from build123d import *

# Parameters (mm, degrees)
EXTRUDE1_DEPTH                      = 19.05
EXTRUDE1_DEPTH_BACK                 = 19.05
F_6_CLEARANCE_HOLE1_D               = 3.7973
F_6_CLEARANCE_HOLE1_DEPTH           = 6.35
F_6_CLEARANCE_HOLE1_TIP             = 1.140824014
F_6_CLEARANCE_HOLE1_ON_FACE_2_D     = 3.7973
F_6_CLEARANCE_HOLE1_ON_FACE_2_DEPTH = 6.35
F_6_CLEARANCE_HOLE1_ON_FACE_2_TIP   = 1.140824014
SKETCH3_W                           = 15.875
SKETCH3_H                           = 9.525
CUT_EXTRUDE1_DEPTH                  = 4.175
CHAMFER1_SIZE                       = 5.08


with BuildPart() as part:
    # Sketch1 → Extrude1 (new body, two sides)
    with BuildSketch(Plane(origin=(0, 0, 0), x_dir=(0, 0, -1), z_dir=(1, 0, 0))) as extrude1_sk:
        Polygon((-3.175, 9.525), (-3.175, -3.175), (9.525, -3.175), (9.525, 0), (0, 0), (0, 9.525), align=None)
    extrude(amount=EXTRUDE1_DEPTH)
    extrude(extrude1_sk.sketch, amount=-EXTRUDE1_DEPTH_BACK)

    # 6 Clearance Hole1
    with Locations(Plane(origin=(6.35, 0, -4.7625), x_dir=(0, 0, 1), z_dir=(0, 1, 0))):
        with Locations((0, 0), (0, -12.7)):
            Hole(F_6_CLEARANCE_HOLE1_D / 2, depth=F_6_CLEARANCE_HOLE1_DEPTH)
            with Locations((0, 0, -(F_6_CLEARANCE_HOLE1_DEPTH + F_6_CLEARANCE_HOLE1_TIP / 2))):  # 118° drill point
                Cone(0, F_6_CLEARANCE_HOLE1_D / 2, F_6_CLEARANCE_HOLE1_TIP, mode=Mode.SUBTRACT)

    # 6 Clearance Hole1 on face 2
    with Locations(Plane(origin=(3.175, 4.826, 0), x_dir=(-1, 0, 0), z_dir=(0, 0, -1))):
        with Locations((0, 0), (-9.525, 0)):
            Hole(F_6_CLEARANCE_HOLE1_ON_FACE_2_D / 2, depth=F_6_CLEARANCE_HOLE1_ON_FACE_2_DEPTH)
            with Locations((0, 0, -(F_6_CLEARANCE_HOLE1_ON_FACE_2_DEPTH + F_6_CLEARANCE_HOLE1_ON_FACE_2_TIP / 2))):  # 118° drill point
                Cone(0, F_6_CLEARANCE_HOLE1_ON_FACE_2_D / 2, F_6_CLEARANCE_HOLE1_ON_FACE_2_TIP, mode=Mode.SUBTRACT)

    # Sketch3 → Cut-Extrude1 (cut, through all)
    with BuildSketch(Plane(origin=(0, 0, 0), x_dir=(-1, 0, 0), z_dir=(0, 0, -1))):
        with Locations((11.1125, 4.7625)):
            Rectangle(SKETCH3_W, SKETCH3_H)
    extrude(amount=-CUT_EXTRUDE1_DEPTH, mode=Mode.SUBTRACT)

    # Chamfer1
    chamfer1_edges = [part.edges().sort_by_distance(p)[0] for p in [
        (19.05, -1.5875, -9.525),
        (-19.05, -1.5875, -9.525),
        (19.05, 9.525, 1.5875),
        (-3.175, 9.525, 1.5875),
    ]]
    chamfer(chamfer1_edges, length=CHAMFER1_SIZE)


solid = part.part
For this review, take the finished solid that the model builds, in its own axes (mm). A direction names the side the tool comes from. Give positions to 0.01 mm unless a question says otherwise; leave off trailing zeros. Loops run counter-clockwise (first coordinate to the right, second up) from the corner with the lowest first, then second, coordinate; pieces in that order, holes last. Notation, with made-up numbers: M 68.5,25.25 L 81.5,25.25 A22 cw 81.5,60.25 Z; hole C 15,-34.75 d4. An arc over 180 degrees is marked long. Put each result on its own line as item: value. Start each with the question number.
(1) Wall thickness on L1, parallel to Y at x = 12.7, z = 1.15 (3 decimals); L2, parallel to X at y = 6.5, z = 0.25 (3 decimals); L3, parallel to Y at x = 14, z = -6.25 (3 decimals): over which ranges is each line inside the solid? List them lowest first.
(2) The part is to be moulded in two halves that separate along X. For faces 1 (the cylindrical face through (4.93, 4.1, 1.61)), 2 (the flat face through (16.546, -1.61, -6.949)), 3 (the flat face through (-3.175, 2, 2)), say which applies: +X half, -X half, draft (parallel to the pull), parting line (faces both ways), or undercut.
(3) Machinability: for faces 4 (the flat face through (8, 5, 0)), 5 (the flat face through (5, 2, 3.175)), which of the approach directions +Z, -Z, +X, -X, +Y, -Y give a long, thin tool a straight path to every point of the face, cutting with its end or side? Answer none if there is none.
(4) Add section C-C, the plane z = -0.75. Write out the cut boundary in (x, y) (3 decimals).
(5) For pin 1 (3 mm diameter, centred on x = 10, y = 5, fed in from -Z); pin 2 (2.5 mm diameter, centred on y = 1.5, z = 2.5, fed in from -X) (3 decimals), all flat-tipped, find the tip position at first contact; note any pin that passes through.
(6) Add section B-B, the plane x = 0. Write out the cut boundary in (y, z) (3 decimals), then the cut area to 3 significant figures.
(7) Add section A-A, the plane x = 12.7. Write out the cut boundary in (y, z) (3 decimals).
(8) Add section D-D, the plane x = -6.35. Write out the cut boundary in (y, z) (3 decimals).
Result:
1. L1: y = -3.175 to 2.927, 6.725 to 9.525
1. L2: x = -1.12 to 2.279, 4.071 to 11.804, 13.596 to 16.995
1. L3: y = -3.175 to 0
2. face 1: undercut
2. face 2: +X half
2. face 3: -X half
3. face 4: -Z, +X, -X, +Y
3. face 5: +Z, +X, -X, +Y, -Y
4. outline: M -19.05,-3.175 L 19.05,-3.175 L 19.05,0 L -19.05,0 Z
5. pin 1: stops at z = 0
5. pin 2: stops at x = -3.175
6. outline: M -3.175,-9.525 L 0,-9.525 L 0,0 L 7.62,0 L 7.62,3.175 L -3.175,3.175 Z
6. area: 64.5 mm^2
7. outline: M -3.175,-9.525 L 0,-9.525 L 0,0 L 2.927,0 L 2.927,3.175 L -3.175,3.175 Z; M 6.725,0 L 9.525,0 L 9.525,3.175 L 6.725,3.175 Z
8. outline: M -3.175,-9.525 L 0,-9.525 L 0,-6.661 L -3.175,-6.661 Z; M -3.175,-2.864 L 0,-2.864 L 0,3.175 L -3.175,3.175 Z
